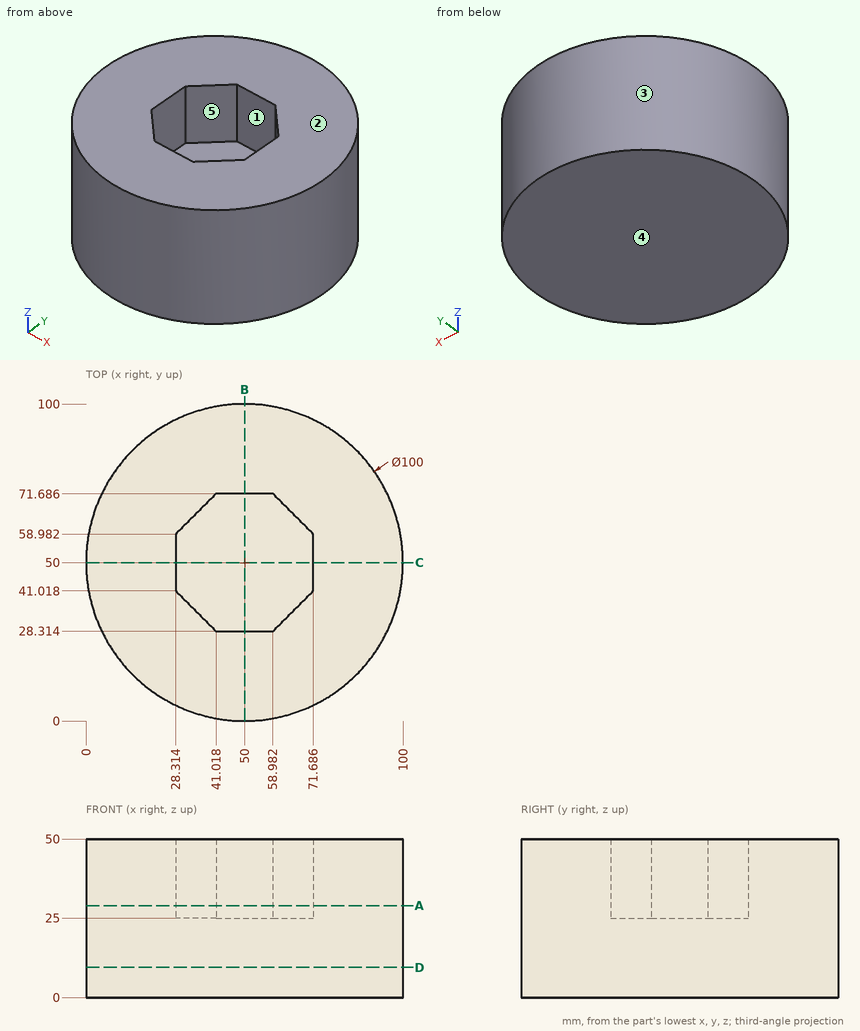
For this review, use the dimensioned drawing (mm, ordinates from the lowest corner) and the shaded views. A direction names the side the tool comes from. Give positions to 0.01 mm unless a question says otherwise; leave off trailing zeros. Order: outer loops, then holes, each group sorted by start corner. A loop starts at its lowest first (then second) coordinate and runs counter-clockwise, first axis right, second up.
1. Add section A-A, the plane z = 29. State the section outline as (x, y) points (1 decimal), then the cut area to 3 significant figures.
Solution:
outline: circle Ø100 at (50, 50); hole (28.3, 41) - (41, 28.3) - (59, 28.3) - (71.7, 41) - (71.7, 59) - (59, 71.7) - (41, 71.7) - (28.3, 59) - close
area: 6,300 mm2
2. To check wall thickness, follow L1, parallel to Z at x = 42, y = 28.5; L2, parallel to X at y = 50.5, z = 21.5; L3, parallel to Y at x = 41, z = 41 (1 decimal). State the ranges of each line that lie inside material, in increasing order.
Solution:
L1: z = 0 to 25
L2: x = 0 to 100
L3: y = 0.8 to 28.3, 71.7 to 99.2
3. Add section D-D, the plane z = 9.5. State the section outline as (x, y) points, then the cut area to 3 significant figures.
Solution:
outline: circle Ø100 at (50, 50)
area: 7,850 mm2
4. Add section B-B, the plane x = 50. State the section outline as (y, z) points (1 decimal), then the cut area to 3 significant figures.
Solution:
outline: (0, 0) - (100, 0) - (100, 50) - (71.7, 50) - (71.7, 25) - (28.3, 25) - (28.3, 50) - (0, 50) - close
area: 3,920 mm2
5. For pin 1 Ø12 at (y, z) = (58.5, 27) entering from +X; pin 2 Ø14.5 at (x, z) = (49.5, 38.5) entering from +Y; pin 3 Ø3 at (x, z) = (49, 27.5) entering from -Y, all flat-tipped, find the tip position at first contact; note any pin that passes through.
Solution:
pin 1: stops at x = 99.94
pin 2: stops at y = 100
pin 3: stops at y = 0
6. Mouldability with a two-part tool opening along Y and no side actions: class the marked faces 1, 2 and 3 as +Y half, -Y half, draft (parallel to the pull), parting line (faces both ways), or undercut.
Solution:
face 1: undercut
face 2: draft
face 3: parting line
7. Tool access review of the marked faces 4 and 5: name each direction out of +Z, -Z, +X, -X, +Y, -Y from which nothing blocks a thin tool from reaching the whole face with its end or side.
Solution:
face 4: -Z, +X, -X, +Y, -Y
face 5: +Z
